```python
from build123d import *

# Parameters (mm, degrees)
F3_DEPTH = 38.079278


with BuildPart() as f1:
    # F0 (on Front) → F1 (revolve)
    with BuildSketch(Plane.XZ):
        with BuildLine():
            Line((11.224204, 30.1519), (19.039139, 30.1519))
            Line((19.039139, 30.1519), (19.039139, 47.066718))
            ThreePointArc((19.039139, 47.066718), (0, 66.105857), (-19.039139, 47.066718))
            Line((-19.039139, 47.066718), (-19.039139, 30.1519))
            Line((-19.039139, 30.1519), (-11.224204, 30.1519))
            Line((-11.224204, 30.1519), (-6.366854, 36.873989))
            Line((-6.366854, 36.873989), (6.366854, 36.873989))
            Line((6.366854, 36.873989), (11.224204, 30.1519))
        make_face()
    revolve(axis=Axis((-0.409778, 0, 0), (1, 0, 0)))

    # F2 (on face) → F3 (cut, through all)
    with BuildSketch(Plane.YZ.offset(19.039139)):
        with BuildLine():
            Line((-6.732479, 37.094571), (-6.732479, 29.390658))
            ThreePointArc((-6.732479, 29.390658), (0, 30.1519), (6.732479, 29.390658))
            Line((6.732479, 29.390658), (6.732479, 37.094571))
            Line((6.732479, 37.094571), (-6.732479, 37.094571))
        make_face()
    extrude(amount=-F3_DEPTH, mode=Mode.SUBTRACT)


solid = f1.part
```
CAD build for the part. Positions are in the model's coordinates, mm. A direction names the side the tool comes from. Round coordinates to 2 decimals unless told otherwise and drop trailing zeros. Write each loop counter-clockwise with the first axis right and the second up, starting at its lowest first coordinate (ties: lowest second). Pieces come first, ordered by that corner, then holes. Notation, with made-up numbers: (-25.75, 7.5) - (-9.75, 7.5) arc R24 cw to (-9.75, 18.5) - close; hole circle Ø4 at (-18.75, 69). An arc over 180 degrees is marked (long way). Write item = value, one per line. Start each with the question number.
Q1. Probe L1, parallel to Y at x = 10, z = -11; L2, parallel to Y at x = -1.5, z = 0; L3, parallel to Z at x = 9.5, y = 15. List the from-to ranges inside material, lowest first. Write a range as from..to.
Q2. Band-saw the part on B-B (y = 0). Give the cut face in (x, z), then the cut area to 3 significant figures.
Q3. Band-saw the part on C-C (x = -15). Give the cut face in (y, z), then the cut area to 3 significant figures.
Q4. Band-saw the part on A-A (z = 0). Give the cut face in (x, y), then the cut area to 3 significant figures.
Q5. Drop flat-ended pins along their axis: pin 1 (5 mm diameter, centred on x = 5.5, z = 2.5, fed in from +Y); pin 2 (2 mm diameter, centred on x = -11.5, z = 15, fed in from +Y); pin 3 (10 mm diameter, centred on y = -4.5, z = 21, fed in from +X); pin 4 (10 mm diameter, centred on x = -8, z = -46.5, fed in from -Y). Give the stop position or say it passes through.
Q6. Band-saw the part on D-D (x = -3.5). Give the cut face in (y, z), then the cut area to 3 significant figures.
Q7. Which spindle directions (+Z, -Z, +X, -X, +Y, -Y) get a long thin tool onto all of the face, cutting with end or side? Do faces 4 (the conical face through (-10.92, -1.266, -30.546)), 5 (the flat face through (0.3, 6.732, 36.6)), 6 (the flat face through (19.039, -1, -31)). Say none if no direction does.
Q8. Mould opens along Z. For faces 1 (the flat face through (0, 0, 37.095)), 2 (the cylindrical face through (15.186, -1.231, -30.127)), 3 (the flat face through (-19.039, 31, -1)) say: pulls with the +Z half, pulls with the -Z half, needs draft (parallel to the pull), parting line crosses it, or undercut.
Answers below:
q1.L1 = -62.3..-29.89, 29.89..62.3
q1.L2 = -66.05..-36.87, 36.87..66.05
q1.L3 = -61.77..-28.87, 28.87..61.77
q2.outline = (-19.04, -47.07) arc R19.04 ccw to (19.04, -47.07) - (19.04, -30.15) - (11.22, -30.15) - (6.37, -36.87) - (-6.37, -36.87) - (-11.22, -30.15) - (-19.04, -30.15) - close; (-19.04, 37.09) - (19.04, 37.09) - (19.04, 47.07) arc R19.04 ccw to (-19.04, 47.07) - close
q2.area = 2,040 mm2
q3.outline = circle Ø117.58 at (0, 0); hole (-6.73, 29.39) arc R30.15 ccw (long way) to (6.73, 29.39) - (6.73, 37.09) - (-6.73, 37.09) - close
q3.area = 7,910 mm2
q4.outline = (-19.04, -47.07) arc R19.04 ccw to (19.04, -47.07) - (19.04, -30.15) - (11.22, -30.15) - (6.37, -36.87) - (-6.37, -36.87) - (-11.22, -30.15) - (-19.04, -30.15) - close; (-19.04, 30.15) - (-11.22, 30.15) - (-6.37, 36.87) - (6.37, 36.87) - (11.22, 30.15) - (19.04, 30.15) - (19.04, 47.07) arc R19.04 ccw to (-19.04, 47.07) - close
q4.area = 2,190 mm2
q5.pin_1 = 65.83
q5.pin_2 = 61.18
q5.pin_3 = through
q5.pin_4 = -49.86
q6.outline = circle Ø131.56 at (0, 0); hole (-6.73, 36.25) arc R36.87 ccw (long way) to (6.73, 36.25) - (6.73, 37.09) - (-6.73, 37.09) - close
q6.area = 9,320 mm2
q7.face_4 = none
q7.face_5 = +X, -X
q7.face_6 = +Z, -Z, +X, +Y, -Y
q8.face_1 = undercut
q8.face_2 = undercut
q8.face_3 = needs draft
